Build history of the part. All positions in model axes, mm. A direction names the side the tool comes from. Round coordinates to 2 decimals unless told otherwise and drop trailing zeros. Loops run counter-clockwise (first coordinate to the right, second up) from the corner with the lowest first, then second, coordinate; pieces in that order, holes last.
from build123d import *

# Parameters (mm, degrees)
F1_DEPTH = 25.4
F3_DEPTH = 12.7
F4_R     = 6.35
F5_DEPTH = 76.201
F6_R     = 6.35


with BuildPart() as f1:
    # F0 (on Front) → F1 (new body, symmetric)
    with BuildSketch(Plane.XZ):
        Polygon((0, 38.1), (0, 0), (76.2, 0), (76.2, 12.7), (50.8, 12.7), (50.8, 25.4), (25.4, 25.4), (25.4, 50.8), (12.7, 50.8), align=None)
    extrude(amount=F1_DEPTH, both=True)

    # F2 (on Front) → F3 (join, symmetric)
    with BuildSketch(Plane.XZ):
        Polygon((25.4, 50.8), (25.4, 25.4), (50.8, 25.4), (50.8, 38.1), (38.1, 38.1), (38.1, 50.8), align=None)
    extrude(amount=F3_DEPTH, both=True)

    # F4 (on face) → F5 (cut, through all)
    with BuildSketch(Plane.YZ.offset(76.2)):
        with Locations((0, 12.7)):
            Circle(F4_R)
    extrude(amount=-F5_DEPTH, mode=Mode.SUBTRACT)

    # F6
    f6_edges = [f1.edges().sort_by_distance(p)[0] for p in [
        (76.2, -25.4, 6.35),
        (76.2, 25.4, 6.35),
    ]]
    fillet(f6_edges, radius=F6_R)


solid = f1.part
(1) Slice it at C-C on x = 49. List the corners of the cut face in (y, z).
Responses:
outline: (-25.4, 0) - (25.4, 0) - (25.4, 25.4) - (12.7, 25.4) - (12.7, 38.1) - (-12.7, 38.1) - (-12.7, 25.4) - (-25.4, 25.4) - close; hole circle Ø12.7 at (0, 12.7)
(2) Pin check, flat tips, straight feed: P1, Ø1.5, axis at x = 34, z = 40.5, coming from the -Y side; P2, Ø6, axis at y = -1.5, z = 19.5, coming from the -X side; P3, Ø14, axis at y = -18.5, z = 41, coming from the +X side; P4, Ø14, axis at x = 43, y = -21, coming from the +Z side. Stop position of each tip, or through.
Responses:
P1: stops at y = -12.7
P2: stops at x = 0
P3: stops at x = 50.8
P4: stops at z = 25.4
(3) Which spindle directions (+Z, -Z, +X, -X, +Y, -Y) get a long thin tool onto all of the face, cutting with end or side? Do faces 5 (the face through (50.8, 0, 25)), 6 (the face through (35, -12.7, 35)), 7 (the face through (35, 12.7, 35)). Say none if no direction does.
Responses:
face 5: +Z, +X, +Y, -Y
face 6: +Z, +X, -Y
face 7: +Z, +X, +Y
(4) Slice it at A-A on y = 0. List the corners of the cut face in (x, z).
Responses:
outline: (0, 0) - (76.2, 0) - (76.2, 6.35) - (0, 6.35) - close; (0, 19.05) - (50.8, 19.05) - (50.8, 38.1) - (38.1, 38.1) - (38.1, 50.8) - (12.7, 50.8) - (0, 38.1) - close
(5) Slice it at D-D on z = 39. List the corners of the cut face in (x, y).
Responses:
outline: (0.9, -25.4) - (25.4, -25.4) - (25.4, -12.7) - (38.1, -12.7) - (38.1, 12.7) - (25.4, 12.7) - (25.4, 25.4) - (0.9, 25.4) - close
(6) Pull direction Z, two halves, no side cores. Call faces 1 (the face through (30.167, 2.93, 7.066)), 2 (the face through (25.4, 19, 38)), 3 (the face through (38, -19, 25.4)), 4 (the face through (38, 0, 0)): +Z half, -Z half, draft (parallel to the pull), parting line (faces both ways), or undercut.
Responses:
face 1: undercut
face 2: draft
face 3: +Z half
face 4: -Z half
(7) Probe line 1 (Z direction, x = 27, y = 0); line 2 (Y direction, x = 47.5, z = 12.7); line 3 (X direction, y = 1.5, z = 24). List the from-to ranges inside material, lowest first.
Responses:
line 1: z = 0 to 6.35, 19.05 to 50.8
line 2: y = -25.4 to -6.35, 6.35 to 25.4
line 3: x = 0 to 50.8
(8) Slice it at B-B on z = 10.5. List the corners of the cut face in (x, y), plus the area to 3 significant figures.
Responses:
outline: (0, -25.4) - (69.85, -25.4) arc R6.35 ccw to (76.2, -19.05) - (76.2, -5.96) - (0, -5.96) - close; (0, 5.96) - (76.2, 5.96) - (76.2, 19.05) arc R6.35 ccw to (69.85, 25.4) - (0, 25.4) - close
area: 2,950 mm2
